Autodesk Inventor part; units mm, degrees
ref_plane "YZ Plane" through (0, 0, 0) normal (1, 0, 0) x (0, 1, 0)
ref_plane "XZ Plane" through (0, 0, 0) normal (0, 1, 0) x (-1, 0, 0)
ref_plane "XY Plane" through (0, 0, 0) normal (0, 0, 1) x (1, 0, 0)
sketch "Szkic1" plane through (0, 0, 0) normal (0, 1, 0) x (-1, 0, 0)
  line L0 (25, 27) -> (-25, 27)
  line L1 (-25, 27) -> (-25, -27)
  line L2 (-25, -27) -> (25, -27)
  line L3 (25, -27) -> (25, 27)
  line L4 (-25, 27) -> (25, -27) construction
  circle A0 centre (15, 21) radius 3
  line L5 (25, 0) -> (-25, 0)
  line L6 (0, 27) -> (0, -27)
  circle A1 centre (15, -21) radius 3
  circle A2 centre (-15, 21) radius 3
  circle A3 centre (-15, -21) radius 3
  line L7 (-25, 27) -> (-30, 27)
  line L8 (-30, 27) -> (-30, -27)
  line L9 (-30, -27) -> (-25, -27)
  line L10 (-25, -27) -> (-25, 27)
  line L11 (0, -14.5) -> (5, -14.5)
  line L12 (5, -14.5) -> (5, -17.5)
  line L13 (5, -17.5) -> (0, -17.5)
  line L14 (0, -17.5) -> (0, -14.5)
  line L15 (0, -14.5) -> (-5, -14.5)
  line L16 (-5, -14.5) -> (-5, -17.5)
  line L17 (-5, -17.5) -> (0, -17.5)
  line L18 (0, 14.5) -> (5, 14.5)
  line L19 (5, 14.5) -> (5, 17.5)
  line L20 (5, 17.5) -> (0, 17.5)
  line L21 (-5, 14.5) -> (-5, 17.5)
  line L22 (-5, 17.5) -> (0, 17.5)
  line L23 (0, 14.5) -> (-5, 14.5)
  line L24 (5, 14.5) -> (5, -14.5)
  line L25 (-5, 14.5) -> (-5, -14.5)
  point P0 (0, 0)
  point P1 (-27.5, 27)
  point P2 (-25, -27)
  point P3 (0, -17.5)
  point P4 (0, 17.5)
  dimension "d0" = 50
  dimension "d5" = 10
  dimension "d7" = 6
  dimension "d8" = 6
  dimension "d9" = 5
  dimension "d10" = 54
  dimension "d12" = 54
  dimension "d21" = 5
  dimension "d22" = 3
  dimension "d26" = 14.5
  dimension "d27" = 50
  dimension "d28" = 36.688
extrude "Wyciągnięcie proste1" add sketch "Szkic1" along normal blind 4 contours L3 L5 L24 L19 L20 L6 L0 | L6 L22 L21 L25 L5 L1 L0 | L3 L2 L6 L13 L12 L24 L5 | L20 L19 L18 L6 | L6 L23 L21 L22 | L24 L11 L6 L5 | L5 L6 L18 L24 | L5 L25 L16 L17 L6 L2 L1 | L6 L5 L25 L23 | L6 L15 L25 L5 | L12 L13 L6 L11 | L17 L16 L15 L6
extrude "Wyciągnięcie proste2" add sketch "Szkic1" along normal blind 70 contours L1 L9 L8 L7
sketch "Szkic3" plane through (-25, 0, 27) normal (0, 0, 1) x (1, 0, 0)
  line L0 (50, 4) -> (50, 70)
  line L1 (50, 9) -> (45, 4)
  line L2 (0, 4) -> (50, 4)
  line L3 (50, 9) -> (57.0711, 9) construction
  point P0 (25, 0)
  dimension "d17" = 135
  dimension "d18" = 5
extrude "Wyciągnięcie proste3" add sketch "Szkic3" against normal blind 54
extrude "Wyciągnięcie proste4" add sketch "Szkic1" along normal blind 42.5 contours L20 L19 L18 L6 | L12 L13 L6 L11
extrude "Wyciągnięcie proste5" add sketch "Szkic1" along normal blind 42.5 contours L24 L11 L6 L5 | L5 L6 L18 L24
extrude "Wyciągnięcie proste6" cut sketch "Szkic1" along normal blind 39.5 contours L24 L11 L6 L5 | L5 L6 L18 L24
extrude "Wyciągnięcie proste7" add sketch "Szkic1" along normal blind 4 contours L24 L11 L6 L5 | L5 L6 L18 L24
sketch "Szkic9" plane through (25, 70, -27) normal (-1, 0, 0) x (0, 0, 1)
  line L0 (0, -66) -> (54, -66)
  line L1 (39.5, -66) -> (39.5, -56)
  line L2 (41.5, -30.5) -> (12.5, -30.5)
  line L3 (41.5, -30.5) -> (41.5, -66)
  line L4 (27, -70) -> (27, 0)
  line L5 (0, 0) -> (54, 0)
  line L6 (14.5, -66) -> (14.5, -56)
  line L7 (39.5, -56) -> (14.5, -56)
  line L8 (39.5, -56) -> (14.5, -56)
  line L9 (14.5, -56) -> (14.5, -66)
  line L10 (14.5, -66) -> (39.5, -66)
  line L11 (39.5, -66) -> (39.5, -56)
  line L12 (39.5, -56) -> (39.5, -30.5)
  line L13 (14.5, -56) -> (14.5, -30.5)
  line L14 (39.5, -40.5) -> (14.5, -40.5)
  line L15 (38, -40.5) -> (16, -40.5)
  line L16 (16, -40.5) -> (16, -30.5)
  line L17 (16, -30.5) -> (38, -30.5)
  line L18 (38, -30.5) -> (38, -40.5)
  point P0 (38, -30.5)
  dimension "d37" = 10
  dimension "d38" = 2
  dimension "d39" = 10
  dimension "d40" = 22
  dimension "d41" = 1.5
extrude "Wyciągnięcie proste8" cut sketch "Szkic9" along normal mid plane 10 contours L0 L4 L7 L1 | L0 L6 L7 L4 | L14 L16 L2 L4 | L4 L2 L18 L14
sketch "Szkic10" plane through (0, 4, -17.5) normal (1, 0, 0) x (0, 0, -1)
  line L0 (-32, 0) -> (-32, 35.5)
  line L1 (-32, 35.5) -> (-3, 35.5)
  line L2 (-3, 35.5) -> (-3, 0)
  line L3 (0, 0) -> (-3, 0)
  line L4 (0, 0) -> (0, 38.5)
  line L5 (-35, 38.5) -> (0, 38.5)
  line L6 (-35, 0) -> (-35, 38.5)
  line L7 (-32, 0) -> (-35, 0)
  point P0 (-17.5, -4)
extrude "Wyciągnięcie proste9" add sketch "Szkic10" along normal up to surface (25 mm away)
properties part number "obudowa_łoż_pion_1" material "Tworzywo sztuczne ABS"
The model under review builds one solid part; all positions refer to its coordinate system, in mm. A direction names the side the tool comes from. Round coordinates to 2 decimals unless told otherwise and drop trailing zeros. Write each loop counter-clockwise with the first axis right and the second up, starting at its lowest first coordinate (ties: lowest second). Pieces come first, ordered by that corner, then holes. Notation, with made-up numbers: M 71,25 L 76,25 A6 cw 76,36 Z; hole C 18,-17.5 d1. An arc over 180 degrees is marked long. Use a Markdown table: item, result. Add a question column.
Q1. The part is to be moulded in two halves that separate along X. For faces 1 (the face through (-12.6, 2, -19.2)), 2 (the face through (25, 24, 0)), 3 (the face through (10, 23, 17.5)), say which applies: pulls with the +X half, pulls with the -X half, needs draft (parallel to the pull), parting line crosses it, or undercut.
Q2. To check wall thickness, follow line 1 (Z direction, x = -15, y = 2); line 2 (Y direction, x = 12.5, z = -14); line 3 (Z direction, x = 9.5, y = 8.5). State the ranges of each line that lie inside material, in increasing order.
Q3. Insertion check: pin 1 (1 mm diameter, centred on x = 18.5, z = 13, fed in from +Y); pin 2 (3 mm diameter, centred on x = -8, z = 0.5, fed in from +Y); pin 3 (8.5 mm diameter, centred on y = 17.5, z = 2, fed in from -X); pin 4 (5.5 mm diameter, centred on x = -15, z = 21, fed in from +Y). Each pin has a flat end and moves straight along its axis. Give the tip position at first contact, or say it passes through.
Q4. We need section D-D, the plane z = 16.5. State the section outline as (x, y) points, plus the area to 4 significant figures.
Q5. Machinability: for faces 4 (the face through (23, 7, 22)), 5 (the face through (13, 39.5, 0)), 6 (the face through (10, 42.5, 0)), 7 (the face through (28, 35, 11)), which of the approach directions +Z, -Z, +X, -X, +Y, -Y give a long, thin tool a straight path to every point of the face, cutting with its end or side? Answer none if there is none.
Q6. We need section A-A, the plane x = 15. State the section outline as (y, z) points.
Q7. We need section B-B, the plane y = 36. State the section outline as (x, z) points, plus the area to 3 significant figures.
Q8. We need section C-C, the plane z = 5.5. State the section outline as (x, y) points, plus the area to 3 significant figures.
Findings below:
| question | item | result |
|---|---|---|
| 1 | face 1 | undercut |
| 1 | face 2 | pulls with the -X half |
| 1 | face 3 | needs draft |
| 2 | line 1 | z = -27 to -24, -18 to 18, 24 to 27 |
| 2 | line 2 | y = 0 to 4, 39.5 to 42.5 |
| 2 | line 3 | z = -17.5 to -14.5, 14.5 to 17.5 |
| 3 | pin 1 | stops at y = 42.5 |
| 3 | pin 2 | stops at y = 4 |
| 3 | pin 3 | stops at x = 25 |
| 3 | pin 4 | passes through |
| 4 | outline | M -25,0 L 30,0 L 30,70 L 25,70 L 25,42.5 L -5,42.5 L -5,4 L -25,4 Z |
| 4 | area | 1,705 mm² |
| 5 | face 4 | +Z, -X, +Y |
| 5 | face 5 | -X |
| 5 | face 6 | +Z, -Z, -X, +Y |
| 5 | face 7 | +X, -X |
| 6 | outline | M 0,-27 L 4,-27 L 4,-24 L 0,-24 Z; M 0,-18 L 4,-18 L 4,-17.5 L 42.5,-17.5 L 42.5,17.5 L 4,17.5 L 4,18 L 0,18 Z; M 0,24 L 4,24 L 4,27 L 0,27 Z; hole M 4,-14.5 L 39.5,-14.5 L 39.5,14.5 L 4,14.5 Z |
| 7 | outline | M -5,-17.5 L 25,-17.5 L 25,-27 L 30,-27 L 30,-11 L 25,-11 L 25,-14.5 L -5,-14.5 Z; M -5,14.5 L 25,14.5 L 25,11 L 30,11 L 30,27 L 25,27 L 25,17.5 L -5,17.5 Z |
| 7 | area | 340 mm² |
| 8 | outline | M -25,0 L 30,0 L 30,4 L -25,4 Z; M -5,39.5 L 30,39.5 L 30,70 L 25,70 L 25,42.5 L -5,42.5 Z; M 25,14 L 30,14 L 30,29.5 L 25,29.5 Z |
| 8 | area | 540 mm² |
